Design review of the part shown in the three views and the two pictorial views. Dimensions are in mm from the part's minimum x, y and z. Give positions to 0.01 mm unless a question says otherwise; leave off trailing zeros. Order: outer loops, then holes, each group sorted by start corner. A loop starts at its lowest first (then second) coordinate and runs counter-clockwise, first axis right, second up.
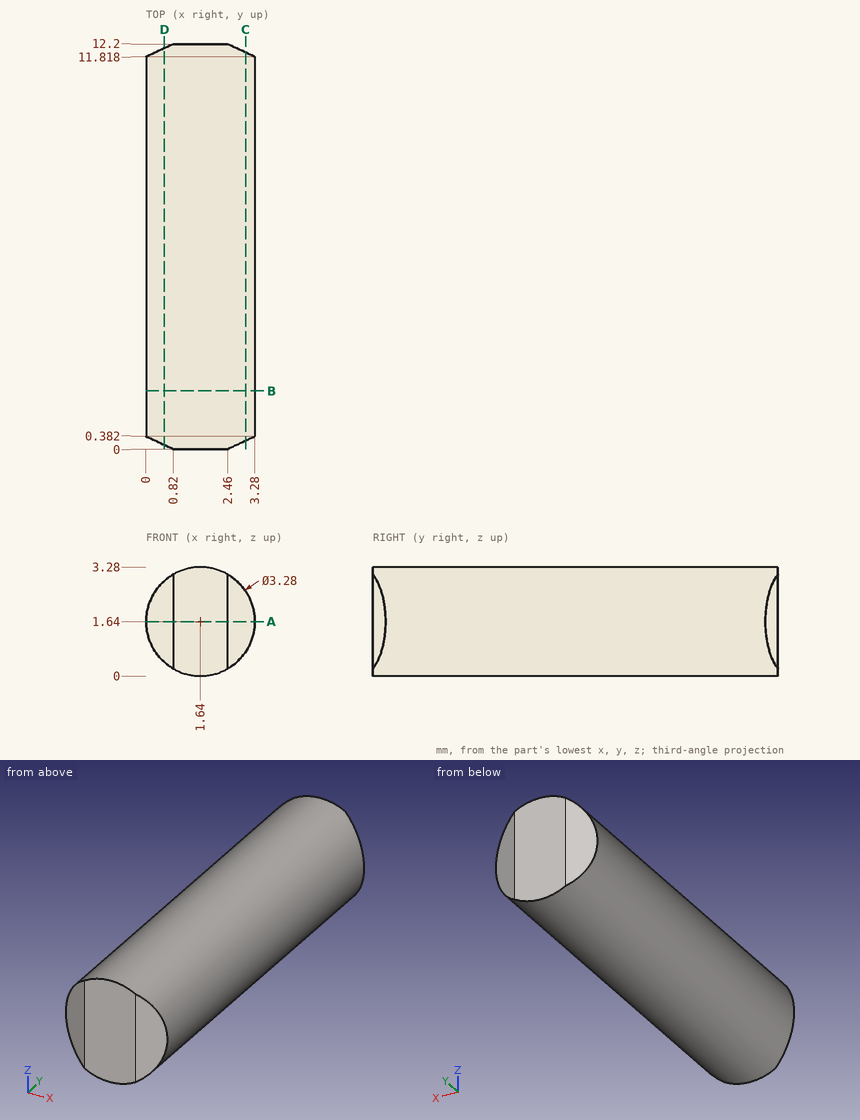
Item 1: Take a section at A-A (z = 1.64). Give the boundary of the cut face in (x, y).
Values found:
outline: (0, 0.38) - (0.82, 0) - (2.46, 0) - (3.28, 0.38) - (3.28, 11.82) - (2.46, 12.2) - (0.82, 12.2) - (0, 11.82) - close
Item 2: Take a section at D-D (x = 0.55). Give the boundary of the cut face in (y, z) (1 decimal), and give its area (3 significant figures).
Values found:
outline: (0.1, 0.4) - (12.1, 0.4) - (12.1, 2.9) - (0.1, 2.9) - close
area: 29.3 mm2
Item 3: Take a section at C-C (x = 3). Give the boundary of the cut face in (y, z).
Values found:
outline: (0.25, 0.72) - (11.95, 0.72) - (11.95, 2.56) - (0.25, 2.56) - close
Item 4: Take a section at B-B (y = 1.75). Give the boundary of the cut face in (x, z).
Values found:
outline: circle Ø3.28 at (1.64, 1.64)
Item 5: For line 1 (Z direction, x = 1.7, y = 10); line 2 (Y direction, x = 0.45, z = 2.6); line 3 (Z direction, x = 2.2, y = 3.5), list the stretches that pass through material, from the lowest coordinate up.
Values found:
line 1: z = 0 to 3.28
line 2: y = 0.17 to 12.03
line 3: z = 0.1 to 3.18
